The listing builds one solid part. Answer for the finished solid, in the listing's coordinates (mm). Round coordinates to 2 decimals unless told otherwise and drop trailing zeros. Order: outer loops, then holes, each group sorted by start corner. A loop starts at its lowest first (then second) coordinate and runs counter-clockwise, first axis right, second up. Notation, with made-up numbers: M 58.25,-27 L 86.25,-27 A24 ccw 86.25,-4 Z; hole C 5,57 d2. An arc over 180 degrees is marked long. Write item = value, one per line. Start each with the question number.
(1) A cutting plane is placed at B-B, the plane x = -51. Determine the outline of the cut face in (y, z), and give its area (3 significant figures).
(2) Straight lines are drawn through the part: probe 1 along Z at (x, y) = (-76, 0.95); probe 2 along Z at (x, y) = (-65.5, 0.6); probe 3 along Z at (x, y) = (-16, 0.4). For each, find the intervals that lie inside material, in ascending order. Write a range as from..to.
(3) This flat-tipped pin is pushed along its axis until it touches: pin 1 (0.5 mm diameter, centred on y = 0.5, z = -63.5, fed in from -X). Where does it stop, or does it pass through?
(4) A cutting plane is placed at C-C, the plane y = 0.8. Count the separate pieces of the cut face and the enclosed holes in it, and give its area (3 significant figures).
(5) For a pull along Z with two mould halves and no side action, classify faces 1 (the face through (-133.314, 0.493, -38.762)), 2 (the face through (-54.476, 0.493, 56.006)), 3 (the face through (-133.314, 0.493, 38.762)) as released by +Z, released by -Z, zero draft, split by the parting line, or undercut.
(6) A cutting plane is placed at A-A, the plane z = 0. Determine the outline of the cut face in (x, y), and give its area (3 significant figures).
(7) A cutting plane is placed at D-D, the plane z = -63. Determine the outline of the cut face in (x, y).
Autodesk Inventor part; units mm, degrees
ref_plane "YZ Plane" through (0, 0, 0) normal (1, 0, 0) x (0, 1, 0)
ref_plane "XZ Plane" through (0, 0, 0) normal (0, 1, 0) x (-1, 0, 0)
ref_plane "XY Plane" through (0, 0, 0) normal (0, 0, 1) x (1, 0, 0)
sketch "Esboço1" plane through (0, 0, 0) normal (0, 1, 0) x (-1, 0, 0)
  line L0 (139.8134, -26.55) -> (126.6305, -51.3208)
  line L1 (139.8134, -26.55) -> (139.8134, 0)
  line L2 (139.8134, -26.55) -> (126.6305, -51.3208)
  circle A0 centre (61.129, 0) radius 23
  circle A1 centre (56.3183, -57.6959) radius 2.5
  circle A2 centre (76.3183, -57.6959) radius 2.5
  circle A3 centre (86.3183, -57.6959) radius 2.5
  circle A4 centre (66.3183, -57.6959) radius 2.5
  line L3 (92.1195, -55.1192) -> (92.1195, -72.3197)
  line L4 (75.8622, -72.3197) -> (92.1195, -72.3197)
  line L5 (36.1237, -90.4148) -> (36.1237, -72.3197)
  line L6 (75.8622, -72.3197) -> (36.1237, -90.4148)
  line L7 (126.6305, -51.3208) -> (92.1195, -51.3208)
  line L8 (92.1195, -51.3208) -> (92.1195, -55.1192)
  line L9 (139.8134, 26.55) -> (126.6305, 51.3208)
  line L10 (139.8134, 26.55) -> (139.8134, 0)
  circle A5 centre (76.3183, 57.6959) radius 2.5
  circle A6 centre (86.3183, 57.6959) radius 2.5
  circle A7 centre (66.3183, 57.6959) radius 2.5
  circle A8 centre (56.3183, 57.6959) radius 2.5
  line L11 (92.1195, 55.1192) -> (92.1195, 72.3197)
  line L12 (75.8622, 72.3197) -> (92.1195, 72.3197)
  line L13 (36.1237, 90.4148) -> (36.1237, 72.3197)
  line L14 (75.8622, 72.3197) -> (36.1237, 90.4148)
  line L15 (126.6305, 51.3208) -> (92.1195, 51.3208)
  line L16 (92.1195, 51.3208) -> (92.1195, 55.1192)
  line L17 (0, 65.2411) -> (0, -65.2411)
  line L18 (36.1237, 72.3197) -> (0, 72.3197)
  line L19 (0, 72.3197) -> (0, 65.2411)
  line L20 (36.1237, -72.3197) -> (0, -72.3197)
  line L21 (0, -72.3197) -> (0, -65.2411)
  point P0 (0, 0)
  dimension "d1" = 46
  dimension "d6" = 130.4821
extrude "Extrusão1" add sketch "Esboço1" along normal blind 1
properties part number "base_1"
Reported:
q1.outline = M 0,-83.64 L 1,-83.64 L 1,-20.65 L 0,-20.65 Z; M 0,20.65 L 1,20.65 L 1,83.64 L 0,83.64 Z
q1.area = 126 mm²
q2.probe_1 = -72.32..-60.18, -55.22..-17.55, 17.55..55.22, 60.18..72.32
q2.probe_2 = -77.04..-60.06, -55.33..-22.58, 22.58..55.33, 60.06..77.04
q2.probe_3 = -72.32..72.32
q3.pin_1 = -92.12
q4.separate_pieces = 1
q4.enclosed_holes = 9
q4.area = 16,800 mm²
q5.face_1 = released by -Z
q5.face_2 = undercut
q5.face_3 = released by +Z
q6.outline = M -139.81,0 L -84.13,0 L -84.13,1 L -139.81,1 Z; M -38.13,0 L 0,0 L 0,1 L -38.13,1 Z
q6.area = 93.8 mm²
q7.outline = M -92.12,0 L 0,0 L 0,1 L -92.12,1 Z
